from build123d import *

# Parameters (mm, degrees)
SKETCH1_R           = 9.061638146
BOSS_EXTRUDE1_DEPTH = 28
FILLET1_R           = 0.75


with BuildPart() as part:
    # Sketch1 → Boss-Extrude1 (new body)
    with BuildSketch(Plane.XY):
        Circle(SKETCH1_R)
        with BuildLine():
            ThreePointArc((3.888321502, -3), (0, 4.911114344), (-3.888321502, -3))
            Line((-3.888321502, -3), (3.888321502, -3))
        make_face(mode=Mode.SUBTRACT)
        with BuildLine():
            ThreePointArc((-4.58615413, -7.815399938), (-5.312879632, -7.340749002), (-5.990857259, -6.798743648))
            ThreePointArc((-5.990857259, -6.798743648), (-10.498546947, -12.514092303), (-17.145581833, -15.480808299))
            Line((-17.145581833, -15.480808299), (-16.970562748, -16.970562748))
            ThreePointArc((-16.970562748, -16.970562748), (-9.561507432, -14.039044926), (-4.58615413, -7.815399938))
        make_face()
        with BuildLine():
            ThreePointArc((-8.769222979, -2.283421609), (-8.947466614, -1.433920183), (-9.04361353, -0.571261944))
            ThreePointArc((-9.04361353, -0.571261944), (-16.272393267, -1.425205789), (-23.070341708, 1.177172655))
            Line((-23.070341708, 1.177172655), (-24, 0))
            ThreePointArc((-24, 0), (-16.688110612, -3.166097125), (-8.769222979, -2.283421609))
        make_face()
        with BuildLine():
            ThreePointArc((-7.815399938, 4.58615413), (-7.340749002, 5.312879632), (-6.798743648, 5.990857259))
            ThreePointArc((-6.798743648, 5.990857259), (-12.514092303, 10.498546947), (-15.480808299, 17.145581833))
            Line((-15.480808299, 17.145581833), (-16.970562748, 16.970562748))
            ThreePointArc((-16.970562748, 16.970562748), (-14.039044926, 9.561507432), (-7.815399938, 4.58615413))
        make_face()
        with BuildLine():
            Line((1.177172655, 23.070341708), (0, 24))
            ThreePointArc((0, 24), (-3.166097125, 16.688110612), (-2.283421609, 8.769222979))
            ThreePointArc((-2.283421609, 8.769222979), (-1.433920183, 8.947466614), (-0.571261944, 9.04361353))
            ThreePointArc((-0.571261944, 9.04361353), (-1.425205789, 16.272393267), (1.177172655, 23.070341708))
        make_face()
        with BuildLine():
            ThreePointArc((16.970562748, 16.970562748), (9.561507432, 14.039044926), (4.58615413, 7.815399938))
            ThreePointArc((4.58615413, 7.815399938), (5.312879632, 7.340749002), (5.990857259, 6.798743648))
            ThreePointArc((5.990857259, 6.798743648), (10.498546947, 12.514092303), (17.145581833, 15.480808299))
            Line((17.145581833, 15.480808299), (16.970562748, 16.970562748))
        make_face()
        with BuildLine():
            ThreePointArc((24, 0), (16.688110612, 3.166097125), (8.769222979, 2.283421609))
            ThreePointArc((8.769222979, 2.283421609), (8.947466614, 1.433920183), (9.04361353, 0.571261944))
            ThreePointArc((9.04361353, 0.571261944), (16.272393267, 1.425205789), (23.070341708, -1.177172655))
            Line((23.070341708, -1.177172655), (24, 0))
        make_face()
        with BuildLine():
            ThreePointArc((16.970562748, -16.970562748), (14.039044926, -9.561507432), (7.815399938, -4.58615413))
            ThreePointArc((7.815399938, -4.58615413), (7.340749002, -5.312879632), (6.798743648, -5.990857259))
            ThreePointArc((6.798743648, -5.990857259), (12.514092303, -10.498546947), (15.480808299, -17.145581833))
            Line((15.480808299, -17.145581833), (16.970562748, -16.970562748))
        make_face()
        with BuildLine():
            ThreePointArc((2.283421609, -8.769222979), (1.433920183, -8.947466614), (0.571261944, -9.04361353))
            ThreePointArc((0.571261944, -9.04361353), (1.425205789, -16.272393267), (-1.177172655, -23.070341708))
            Line((-1.177172655, -23.070341708), (0, -24))
            ThreePointArc((0, -24), (3.166097125, -16.688110612), (2.283421609, -8.769222979))
        make_face()
    extrude(amount=BOSS_EXTRUDE1_DEPTH)

    # Fillet1
    fillet1_edges = [part.edges().sort_by_distance(p)[0] for p in [
        (-17.058072291, -16.225685524, 28),
        (-0.588586328, -23.535170854, 28),
        (16.225685524, -17.058072291, 28),
        (23.535170854, -0.588586328, 28),
        (16.225685524, -17.058072291, 0),
        (-0.588586328, -23.535170854, 0),
        (-17.058072291, -16.225685524, 0),
        (-23.535170854, 0.588586328, 0),
        (-16.225685524, 17.058072291, 0),
        (17.058072291, 16.225685524, 28),
        (0.588586328, 23.535170854, 0),
        (17.058072291, 16.225685524, 0),
        (23.535170854, -0.588586328, 0),
        (16.970562748, -16.970562748, 14),
        (15.480808299, -17.145581833, 14),
        (0, -24, 14),
        (-1.177172655, -23.070341708, 14),
        (0.588586328, 23.535170854, 28),
        (-16.970562748, -16.970562748, 14),
        (-17.145581833, -15.480808299, 14),
        (-24, 0, 14),
        (-23.070341708, 1.177172655, 14),
        (-16.970562748, 16.970562748, 14),
        (-15.480808299, 17.145581833, 14),
        (0, 24, 14),
        (1.177172655, 23.070341708, 14),
        (16.970562748, 16.970562748, 14),
        (17.145581833, 15.480808299, 14),
        (24, 0, 14),
        (23.070341708, -1.177172655, 14),
        (-16.225685524, 17.058072291, 28),
        (-23.535170854, 0.588586328, 28),
    ]]
    fillet(fillet1_edges, radius=FILLET1_R)


solid = part.part
The listing builds one solid part. Answer for the finished solid, in the listing's coordinates (mm). A direction names the side the tool comes from. Round coordinates to 2 decimals unless told otherwise and drop trailing zeros. Loops run counter-clockwise (first coordinate to the right, second up) from the corner with the lowest first, then second, coordinate; pieces in that order, holes last. Notation, with made-up numbers: M 59,-31.75 L 64,-31.75 A17 cw 64,-20.75 Z; hole C 62.5,79.5 d8. An arc over 180 degrees is marked long. Write each question's results on one line, items separated by ' | '. Start each with the question number.
1) Each of these flat-tipped pins is pushed along its axis until it touches: pin 1 (3 mm diameter, centred on y = -15, z = 20.5, fed in from +X); pin 2 (1 mm diameter, centred on x = 11.5, z = 19, fed in from +Y); pin 3 (4 mm diameter, centred on x = -13.5, y = -5.5, fed in from -Z); pin 4 (1 mm diameter, centred on x = -13.5, z = 16.5, fed in from -Y). Where does it stop, or does it pass through?
2) Find section B-B on x = -19. Write down the section's boundary in (y, z), plus the area to 3 significant figures.
3) Which of the six approach directions +Z, -Z, +X, -X, +Y, -Y give full straight-line access (tool end or side, diameter ignored) to faces 1 (the cylindrical face through (-3.206, 16.404, 13.804)), 2 (the cylindrical face through (10.159, 12.242, 13.804)), 3 (the cylindrical face through (-10.159, -12.242, 13.804)), 4 (the cylindrical face through (-0.42, -23.27, 0.14)), 5 (the cylindrical face through (-23.27, 0.42, 0.14))?
4) Determine the mould class of faces 6 (the cylindrical face through (-12.242, 10.159, 13.804)), 7 (the cylindrical face through (-0.42, -23.27, 27.86)), 8 (the cylindrical face through (0.42, 23.27, 27.86)) for opening direction X: pulls with the +X half, pulls with the -X half, needs draft (parallel to the pull), parting line crosses it, or undercut.
5) Straight lines are drawn through the part: probe 1 along X at (y, z) = (14.5, 20.25); probe 2 along Y at (x, z) = (10, 14.5); probe 3 along Y at (x, z) = (10.5, 16.25). For each, find the intervals that lie inside material, in ascending order.
6) Find section C-C on x = 18. Write down the section's boundary in (y, z).
7) Find section A-A on x = 11. Write down the section's boundary in (y, z).
Final values:
1) pin 1: x = 16.87 | pin 2: y = 15.52 | pin 3: through | pin 4: y = -16.32
2) outline: M -2.64,0 L -0.83,0 L -0.83,28 L -2.64,28 Z | area: 50.7 mm²
3) face 1: +Z, -Z | face 2: +Z, -Z, +X | face 3: +Z, -Z, -X | face 4: -Z, -X, -Y | face 5: -Z, -X, +Y
4) face 6: undercut | face 7: pulls with the -X half | face 8: pulls with the +X half
5) probe 1: -16.47 to -14.75, -3.34 to -1.54, 10.22 to 13.87 | probe 2: -7.95 to -5.76, 0.89 to 2.7, 12.11 to 14.35 | probe 3: -8.37 to -6.1, 1.04 to 2.84, 12.52 to 14.68
6) outline: M 1.11,0 L 2.91,0 L 2.91,28 L 1.11,28 Z
7) outline: M -8.83,0 L -6.47,0 L -6.47,28 L -8.83,28 Z; M 1.16,0 L 2.96,0 L 2.96,28 L 1.16,28 Z; M 12.89,0 L 14.98,0 L 14.98,28 L 12.89,28 Z
